Could you check a few things on this model? Use its own coordinates, in mm. A direction names the side the tool comes from. Coordinates: 2 decimals unless noted, no trailing zeros. Loops run counter-clockwise (first coordinate to the right, second up) from the corner with the lowest first, then second, coordinate; pieces in that order, holes last. Notation, with made-up numbers: (-30, 68.25) -> (26, 68.25) arc R23 cw to (26, 99.25) -> close; hole circle Ø11 at (25, -25). An arc over 180 degrees is marked (long way). One line per question, with ' | ' between items.
```python
from build123d import *

# Parameters (mm, degrees)
SKETCH_1_R          = 1.6
EXTRUDE_1_DEPTH     = 154
SKETCH_5_R          = 3.05
CUT_EXTRUDE_3_DEPTH = 222.645137515
SKETCH_6_W          = 125
SKETCH_6_H          = 148
CUT_EXTRUDE_5_DEPTH = 126
SKETCH_7_R          = 1.6
CUT_EXTRUDE_6_DEPTH = 119
FILLET_1_R          = 10


with BuildPart() as part:
    # 草图1 → 凸台-拉伸1 (new body)
    with BuildSketch(Plane.XY):
        Polygon((3.292616486, 24.576402747), (3.292616486, -25.423597253), (-121.707383514, -25.423597253), (-121.707383514, 14.576402747), (-56.707383514, 26.515067344), (-56.707383514, 102.946004208), (-6.707383514, 102.946004208), (-6.707383514, 24.576402747), align=None)
        with Locations((-6.707383514, -10.423597253)):
            Circle(SKETCH_1_R, mode=Mode.SUBTRACT)
        with Locations((-6.707383514, -0.423597253)):
            Circle(SKETCH_1_R, mode=Mode.SUBTRACT)
        with Locations((-6.707383514, 9.576402747)):
            Circle(SKETCH_1_R, mode=Mode.SUBTRACT)
        with Locations((-6.707383514, 19.576402747)):
            Circle(SKETCH_1_R, mode=Mode.SUBTRACT)
    extrude(amount=EXTRUDE_1_DEPTH)

    # 草图5 → 切除-拉伸3 (cut, through all)
    with BuildSketch(Plane.XY.offset(154)):
        with Locations((-113.707383514, 9.576402747)):
            Circle(SKETCH_5_R)
    extrude(amount=-CUT_EXTRUDE_3_DEPTH, mode=Mode.SUBTRACT)

    # 草图6 → 切除-拉伸5 (cut)
    with BuildSketch(Plane.XZ.offset(25.423597253)):
        with Locations((-59.207383514, 77)):
            Rectangle(SKETCH_6_W, SKETCH_6_H)
    extrude(amount=-CUT_EXTRUDE_5_DEPTH, mode=Mode.SUBTRACT)

    # 草图7 → 切除-拉伸6 (cut)
    with BuildSketch(Plane(origin=(0, 102.946004208, 0), x_dir=(1, 0, 0), z_dir=(0, 1, 0))):
        with Locations(Location((-51.707383514, -82, 0), (0, 0, 270))):
            Circle(SKETCH_7_R)
        with Locations(Location((-51.707383514, -72, 0), (0, 0, 270))):
            Circle(SKETCH_7_R)
    extrude(amount=-CUT_EXTRUDE_6_DEPTH, mode=Mode.SUBTRACT)

    # 圆角1
    fillet_1_edges = [part.edges().sort_by_distance(p)[0] for p in [
        (-6.707383514, 24.576402747, 1.5),
        (-6.707383514, 24.576402747, 152.5),
    ]]
    fillet(fillet_1_edges, radius=FILLET_1_R - 0.0001)  # a hair under: the kernel refuses the full size


solid = part.part
```
Q1. For faces 4 (the face through (-56.707, 101, 42)), 5 (the face through (-46, 23, 151)), 6 (the face through (-44, 25, 0)), which set-ups out of +Z, -Z, +X, -X, +Y, -Y let a thin tool reach every point of the face, with its end or its side?
Values follow:
face 4: +Z, -Z, -X, +Y | face 5: +X, -X, -Y | face 6: -Z, +X, -X, +Y, -Y
Q2. Please list where these lines run through material, in increasing order: L1, parallel to Z at x = -4, y = -6.5; L2, parallel to Y at x = -21.5, z = 96.5. Write a range as [from, to].
Values follow:
L1: z = [0, 3], [151, 154] | L2: y = [100.58, 102.95]
Q3. For pin 1 (5 mm diameter, centred on x = -51.71, z = 72, fed in from -Y), with a flat end and sliding along its axis, tell me the tip position at first contact or that it passes through.
Values follow:
pin 1: stops at y = 100.58
Q4. We'd pull the mould along Y, two halves only. Please class faces 1 (the face through (-3.856, 27.583, 152.521)), 2 (the face through (-6.707, 102, 42)), 3 (the face through (-110.8, 10.5, 1.5)): released by +Y, released by -Y, zero draft, split by the parting line, or undercut.
Values follow:
face 1: released by +Y | face 2: zero draft | face 3: undercut
Q5. Imagine slicing it at C-C on z = 35. Write out the boundary of the cut face in (x, y).
Values follow:
outline: (-56.71, 100.58) -> (-6.71, 100.58) -> (-6.71, 102.95) -> (-56.71, 102.95) -> close
Q6. Imagine slicing it at B-B on x = -61.5. Write out the boundary of the cut face in (y, z).
Values follow:
outline: (-25.42, 0) -> (25.63, 0) -> (25.63, 3) -> (-25.42, 3) -> close; (-25.42, 151) -> (25.63, 151) -> (25.63, 154) -> (-25.42, 154) -> close
Q7. Imagine slicing it at A-A on y = 73.5. Write out the boundary of the cut face in (x, z).
Values follow:
outline: (-56.71, 0) -> (-6.71, 0) -> (-6.71, 3) -> (-56.71, 3) -> close; (-56.71, 151) -> (-6.71, 151) -> (-6.71, 154) -> (-56.71, 154) -> close
